Verification items for the finished model (mm, model axes). Face numbers are marked on the shaded views. A direction names the side the tool comes from. Coordinates: 2 decimals unless noted, no trailing zeros. Order: outer loops, then holes, each group sorted by start corner. A loop starts at its lowest first (then second) coordinate and runs counter-clockwise, first axis right, second up. Notation, with made-up numbers: M 24,32 L 29,32 A18 cw 29,52 Z; hole C 23.5,-20 d10. An arc over 180 degrees is marked long. Answer as a JSON object with one key per item and string values. Group by question number.
(1) Cross-section at D-D (x = -5). Enter the section's corners in (y, z).
(2) Gauge pin test, flat ends, axial feed: pin 1 Ø4 at (y, z) = (-8.5, 28) entering from -X; pin 2 Ø4 at (y, z) = (-27, 12.5) entering from -X; pin 3 Ø8 at (y, z) = (0, 27.5) entering from -X; pin 4 Ø4 at (x, z) = (-12, 13) entering from +Y. Record the tip position at first contact, or that the pin passes through.
(3) Material ranges on line 1 (Y direction, x = -53.5, z = 0); line 2 (Z direction, x = -51, y = 1); line 3 (Y direction, x = -35.5, z = -11.5), recorded low to high.
(4) Cross-section at C-C (x = -50.5). Enter the section's corners in (y, z), plus the area to 3 significant figures.
(5) Access from +Z, -Z, +X, -X, +Y, -Y to the whole of each face (thin tool, end or side, straight path). Record for the marked faces 1, 2 and 3.
from build123d import *

# Parameters (mm, degrees)
SKETCH3_R                       = 25
SKETCH3_R_2                     = 20
BOSS_EXTRUDE2_DEPTH             = 35
FILLET1_R                       = 5
BOSS_EXTRUDE1_REACH             = 113.924
SKETCH2_R                       = 5
BOSS_EXTRUDE1_DIRECTION_2_DEPTH = 3


with BuildPart() as part:
    # Sketch1 → Revolve1 (revolve)
    with BuildSketch(Plane.XY, mode=Mode.PRIVATE) as revolve1_sk:
        with BuildLine():
            Line((-10.818024311, 35), (-38.301363812, 35))
            Line((-38.301363812, 35), (-38.301363812, 20))
            Line((-38.301363812, 20), (11.698636188, 20))
            Line((11.698636188, 20), (11.698636188, 22))
            Line((11.698636188, 22), (4.613699697, 26.09048999))
            Line((4.613699697, 26.09048999), (3.863699697, 24.791451884))
            ThreePointArc((3.863699697, 24.791451884), (0.448636188, 23.876388375), (-0.466427322, 27.291451884))
            Line((-0.466427322, 27.291451884), (0.283572678, 28.59048999))
            Line((0.283572678, 28.59048999), (-10.818024311, 35))
        make_face()
    revolve(revolve1_sk.sketch.rotate(Axis((-10.823091425, 0, 0), (1, 0, 0)), 90), axis=Axis((-10.823091425, 0, 0), (1, 0, 0)))

    # Sketch3 → Boss-Extrude2 (add)
    with BuildSketch(Plane.ZY.offset(38.301363812)):
        with Locations(Location((0, 0, 0), (0, 0, 180))):
            Circle(SKETCH3_R)
        Circle(SKETCH3_R_2, mode=Mode.SUBTRACT)
    extrude(amount=BOSS_EXTRUDE2_DEPTH)

    # Fillet1
    fillet1_edges = [part.edges().sort_by_distance(p)[0] for p in [
        (-38.301363812, 0, 25),
        (-38.301363812, 0, -35),
    ]]
    fillet(fillet1_edges, radius=FILLET1_R - 0.0001)  # a hair under: the kernel refuses the full size

    # Sketch2 → Boss-Extrude1 (add, up to next)
    with BuildSketch(Plane(origin=(0, 42, 0), x_dir=(1, 0, 0), z_dir=(0, 1, 0)), mode=Mode.PRIVATE) as boss_extrude1_sk1:
        with Locations(Location((-22.059694062, 0, 0), (0, 0, 90))):
            Circle(SKETCH2_R)
    boss_extrude1_tool1 = extrude(boss_extrude1_sk1.sketch, amount=-BOSS_EXTRUDE1_REACH, mode=Mode.PRIVATE) - part.part
    boss_extrude1 = boss_extrude1_tool1.solids().sort_by_distance((-22.059694, 42, 0))[0]
    add(boss_extrude1)

    # Sketch2 → Boss-Extrude1 direction 2 (add)
    with BuildSketch(Plane(origin=(0, 42, 0), x_dir=(1, 0, 0), z_dir=(0, 1, 0))):
        with Locations(Location((-22.059694062, 0, 0), (0, 0, 90))):
            Circle(SKETCH2_R)
    boss_extrude1_direction_2 = extrude(amount=BOSS_EXTRUDE1_DIRECTION_2_DEPTH)

    # Mirror1: Boss-Extrude1, Boss-Extrude1 direction 2 across plane
    add(boss_extrude1.mirror(Plane.ZX))
    add(boss_extrude1_direction_2.mirror(Plane.ZX))


solid = part.part
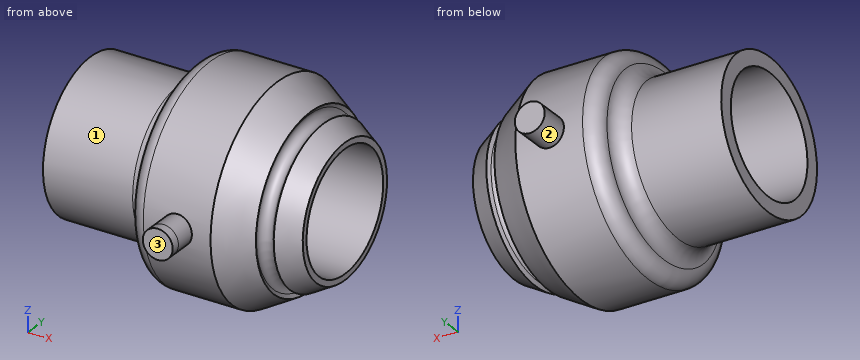
Taken from the geometry:
{
 "1": {"outline": "C 0,0 d63.28; hole C 0,0 d40"},
 "2": {"pin 1": "stops at x = -39.12", "pin 2": "stops at x = -38.83", "pin 3": "stops at x = -73.3", "pin 4": "stops at y = 33.23"},
 "3": {"line 1": "y = -25 to -20, 20 to 25", "line 2": "z = -24.98 to -19.97, 19.97 to 24.98", "line 3": "y = -32.52 to -16.36, 16.36 to 32.52"},
 "4": {"outline": "C 0,0 d50; hole C 0,0 d40", "area": "707 mm²"},
 "5": {"face 1": "-X", "face 2": "+Y", "face 3": "+Z, -Z, +X, -X, -Y"}
}
